Work out the finished part from the listing and answer in its coordinate system (mm). Face numbers are marked on the shaded views. A direction names the side the tool comes from. Coordinates: 2 decimals unless noted, no trailing zeros. Loops run counter-clockwise (first coordinate to the right, second up) from the corner with the lowest first, then second, coordinate; pieces in that order, holes last. Notation, with made-up numbers: (85.25, 68.25) - (89.25, 68.25) arc R38 ccw to (89.25, 106.25) - close; hole circle Ø4 at (55.25, 14.25). An arc over 180 degrees is marked (long way). Write each question's results on one line, items separated by ' | '. Start each with the question number.
1. Which of the six approach directions +Z, -Z, +X, -X, +Y, -Y give full straight-line access (tool end or side, diameter ignored) to the marked faces 5, 6 and 7?
2. Each of these flat-tipped pins is pushed along its axis until it touches: P1, Ø4, axis at x = 10.5, y = 27, coming from the -Z side; P2, Ø6.5, axis at x = 3.5, y = 4, coming from the +Z side; P3, Ø4, axis at x = 0, z = 7, coming from the -Y side; P4, Ø3, axis at y = 14.5, z = 1, coming from the -X side. Where does it stop, or does it pass through?
3. A cutting plane is placed at B-B on y = 4. Determine the outline of the cut face in (x, z), then the cut area to 3 significant figures.
4. Determine the mould class of the marked faces 1, 2, 3 and 4 for opening direction X: released by +X, released by -X, zero draft, split by the parting line, or undercut.
5. A cutting plane is placed at C-C on z = 12. Determine the outline of the cut face in (x, y) (3 decimals), then the cut area to 3 significant figures.
6. A cutting plane is placed at D-D on x = 19. Determine the outline of the cut face in (y, z), then the cut area to 3 significant figures.
7. A cutting plane is placed at A-A on z = 7. Determine the outline of the cut face in (x, y).
8. Find the intervals of material crossed by line 1 along Y through (x, z) = (20, 2.75); line 2 along X through (y, z) = (35, 12.5); line 3 along X through (y, z) = (34.5, 12), in increasing order. Write a range as [from, to].
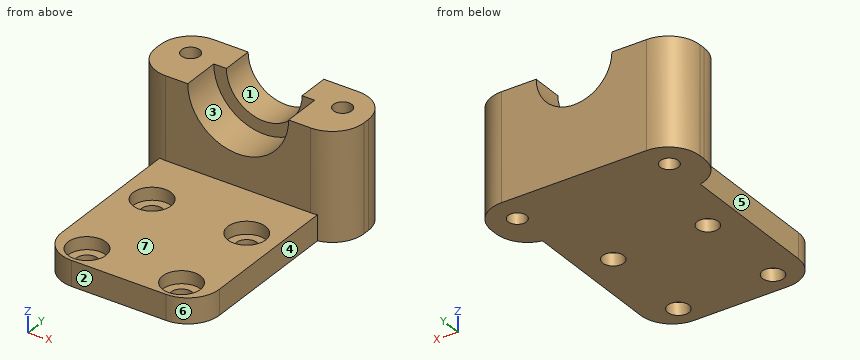
from build123d import *

# Parameters (mm, degrees)
F0_W      = 25
F0_H      = 38.5
F1_DEPTH  = 4
F2_R      = 1.675
F3_DEPTH  = 25
F4_W      = 25
F4_H      = 11
F5_DEPTH  = 13
F7_DEPTH  = 6
F8_R      = 8
F9_DEPTH  = 6
F2_R_2    = 3
F10_DEPTH = 2
F11_W     = 11
F11_H     = 17
F12_DEPTH = 4
F13_R     = 5
F14_W     = 11
F14_H     = 17
F15_DEPTH = 4
F16_DEPTH = 2
F17_R     = 1.45
F18_DEPTH = 25
F19_R     = 5
F20_DEPTH = 25


with BuildPart() as f1:
    # F0 (on Top) → F1 (new body)
    with BuildSketch(Plane.XY):
        with Locations((12.5, 19.25)):
            Rectangle(F0_W, F0_H)
    extrude(amount=F1_DEPTH)

    # F2 (on face) → F3 (cut)
    with BuildSketch(Plane.XY.offset(4)):
        with BuildLine():
            ThreePointArc((3.325, 18.5605346784), (5, 16.8855346784), (6.675, 18.5605346784))
            ThreePointArc((6.675, 18.5605346784), (5, 20.2355346784), (3.325, 18.5605346784))
        make_face()
        with Locations((20, 18.5605346784)):
            Circle(F2_R)
        with Locations((20, 3.5605346784)):
            Circle(F2_R)
        with Locations((5, 3.5605346784)):
            Circle(F2_R)
    extrude(amount=-F3_DEPTH, mode=Mode.SUBTRACT)

    # F4 (on face) → F5 (join)
    with BuildSketch(Plane.XY.offset(4)):
        with Locations((12.5, 33)):
            Rectangle(F4_W, F4_H)
    extrude(amount=F5_DEPTH)

    # F6 (on face) → F7 (cut)
    with BuildSketch(Plane(origin=(0, 38.5, 0), x_dir=(-1, 0, 0), z_dir=(0, 1, 0))):
        with BuildLine():
            ThreePointArc((-18.5, 17), (-12.5, 11), (-6.5, 17))
            Line((-6.5, 17), (-18.5, 17))
        make_face()
    extrude(amount=-F7_DEPTH, mode=Mode.SUBTRACT)

    # F8 (on face) → F9 (cut)
    with BuildSketch(Plane.XZ.offset(-27.5)):
        with Locations((12.5, 17)):
            Circle(F8_R)
    extrude(amount=-F9_DEPTH, mode=Mode.SUBTRACT)

    # F2 (on face) → F10 (cut)
    with BuildSketch(Plane.XY.offset(4)):
        with BuildLine():
            ThreePointArc((8, 18.5605346784), (5, 21.5605346784), (2, 18.5605346784))
            ThreePointArc((2, 18.5605346784), (5, 15.5605346784), (8, 18.5605346784))
        make_face()
        with BuildLine():
            ThreePointArc((3.325, 18.5605346784), (5, 20.2355346784), (6.675, 18.5605346784))
            ThreePointArc((6.675, 18.5605346784), (5, 16.8855346784), (3.325, 18.5605346784))
        make_face(mode=Mode.SUBTRACT)
        with Locations((20, 18.5605346784)):
            Circle(F2_R_2)
        with Locations((20, 18.5605346784)):
            Circle(F2_R, mode=Mode.SUBTRACT)
        with Locations((20, 3.5605346784)):
            Circle(F2_R_2)
        with Locations((20, 3.5605346784)):
            Circle(F2_R, mode=Mode.SUBTRACT)
        with Locations((5, 3.5605346784)):
            Circle(F2_R_2)
        with Locations((5, 3.5605346784)):
            Circle(F2_R, mode=Mode.SUBTRACT)
    extrude(amount=-F10_DEPTH, mode=Mode.SUBTRACT)

    # F11 (on face) → F12 (join)
    with BuildSketch(Plane(origin=(0, 0, 0), x_dir=(0, -1, 0), z_dir=(-1, 0, 0))):
        with Locations((-33, 8.5)):
            Rectangle(F11_W, F11_H)
    extrude(amount=F12_DEPTH)

    # F13
    f13_edges = [f1.edges().sort_by_distance(p)[0] for p in [
        (0, 0, 2),
        (25, 0, 2),
    ]]
    fillet(f13_edges, radius=F13_R)

    # F14 (on face) → F15 (join)
    with BuildSketch(Plane.YZ.offset(25)):
        with Locations((33, 8.5)):
            Rectangle(F14_W, F14_H)
    extrude(amount=F15_DEPTH)

    # F14 (on face) → F16 (join)
    with BuildSketch(Plane.YZ.offset(25)):
        with Locations((33, 8.5)):
            Rectangle(F14_W, F14_H)
    extrude(amount=F16_DEPTH)

    # F17 (on face) → F18 (cut)
    with BuildSketch(Plane.XY.offset(17)):
        with Locations((0.45, 34.05)):
            Circle(F17_R)
        with Locations((24.55, 34.05)):
            Circle(F17_R)
    extrude(amount=-F18_DEPTH, mode=Mode.SUBTRACT)

    # F19
    f19_edges = [f1.edges().sort_by_distance(p)[0] for p in [
        (-4, 38.5, 8.5),
        (-4, 27.5, 8.5),
        (29, 27.5, 8.5),
        (29, 38.5, 8.5),
    ]]
    fillet(f19_edges, radius=F19_R)

    # F2 (on face) → F20 (cut)
    with BuildSketch(Plane.XY.offset(4)):
        with BuildLine():
            ThreePointArc((8, 18.5605346784), (5, 21.5605346784), (2, 18.5605346784))
            ThreePointArc((2, 18.5605346784), (5, 15.5605346784), (8, 18.5605346784))
        make_face()
        with BuildLine():
            ThreePointArc((3.325, 18.5605346784), (5, 20.2355346784), (6.675, 18.5605346784))
            ThreePointArc((6.675, 18.5605346784), (5, 16.8855346784), (3.325, 18.5605346784))
        make_face(mode=Mode.SUBTRACT)
        with Locations((20, 18.5605346784)):
            Circle(F2_R_2)
        with Locations((20, 18.5605346784)):
            Circle(F2_R, mode=Mode.SUBTRACT)
        with BuildLine():
            ThreePointArc((3.325, 18.5605346784), (5, 16.8855346784), (6.675, 18.5605346784))
            ThreePointArc((6.675, 18.5605346784), (5, 20.2355346784), (3.325, 18.5605346784))
        make_face()
        with Locations((20, 18.5605346784)):
            Circle(F2_R)
    extrude(amount=F20_DEPTH, mode=Mode.SUBTRACT)


solid = f1.part
Values:
1) face 5: +Z, -Z, -X, -Y | face 6: +Z, -Z, +X, -Y | face 7: +Z, +X, -X, -Y
2) P1: z = 0 | P2: z = 4 | P3: y = 27.5 | P4: x = 0
3) outline: (0.1, 0) - (3.38, 0) - (3.38, 2) - (2.03, 2) - (2.03, 4) - (0.1, 4) - close; (6.62, 0) - (18.38, 0) - (18.38, 2) - (17.03, 2) - (17.03, 4) - (7.97, 4) - (7.97, 2) - (6.62, 2) - close; (21.62, 0) - (24.9, 0) - (24.9, 4) - (22.97, 4) - (22.97, 2) - (21.62, 2) - close | area: 62.5 mm^2
4) face 1: undercut | face 2: zero draft | face 3: undercut | face 4: released by +X
5) outline: (-4, 32.5) arc R5 ccw to (1, 27.5) - (6.255, 27.5) - (6.255, 33.5) - (9.183, 33.5) - (9.183, 38.5) - (1, 38.5) arc R5 ccw to (-4, 33.5) - close; (15.817, 33.5) - (18.745, 33.5) - (18.745, 27.5) - (24, 27.5) arc R5 ccw to (29, 32.5) - (29, 33.5) arc R5 ccw to (24, 38.5) - (15.817, 38.5) - close; hole circle Ø2.9 at (0.45, 34.05); hole circle Ø2.9 at (24.55, 34.05) | area: 220 mm^2
6) outline: (0, 0) - (2.22, 0) - (2.22, 2) - (0.73, 2) - (0.73, 4) - (0, 4) - close; (4.9, 0) - (17.22, 0) - (17.22, 2) - (15.73, 2) - (15.73, 4) - (6.39, 4) - (6.39, 2) - (4.9, 2) - close; (19.9, 0) - (38.5, 0) - (38.5, 17) - (33.5, 17) - (33.5, 12.34) - (27.5, 12.34) - (27.5, 4) - (21.39, 4) - (21.39, 2) - (19.9, 2) - close | area: 236 mm^2
7) outline: (-4, 32.5) arc R5 ccw to (1, 27.5) - (24, 27.5) arc R5 ccw to (29, 32.5) - (29, 33.5) arc R5 ccw to (24, 38.5) - (1, 38.5) arc R5 ccw to (-4, 33.5) - close; hole circle Ø2.9 at (0.45, 34.05); hole circle Ø2.9 at (24.55, 34.05)
8) line 1: [0, 0.56], [6.56, 15.56], [21.56, 38.5] | line 2: [-3.77, -0.65], [1.55, 8.53], [16.47, 23.45], [25.65, 28.77] | line 3: [-3.9, -0.93], [1.83, 9.18], [15.82, 23.17], [25.93, 28.9]
